```python
from build123d import *

# Parameters (mm, degrees)
SKETCH1_W           = 50.8
SKETCH1_H           = 25.4
BOSS_EXTRUDE1_DEPTH = 6.35
SKETCH2_R           = 3.5
CUT_EXTRUDE1_DEPTH  = 6.35


with BuildPart() as part:
    # Sketch1 → Boss-Extrude1 (new body)
    with BuildSketch(Plane.XY):
        with Locations((25.4, 12.7)):
            Rectangle(SKETCH1_W, SKETCH1_H)
    extrude(amount=BOSS_EXTRUDE1_DEPTH)

    # Sketch2 → Cut-Extrude1 (cut)
    with BuildSketch(Plane.XY.offset(6.35)):
        with Locations((12.7, 12.7)):
            Circle(SKETCH2_R)
        with Locations((38.1, 12.7)):
            Circle(SKETCH2_R)
    extrude(amount=-CUT_EXTRUDE1_DEPTH, mode=Mode.SUBTRACT)


solid = part.part
```
CAD build for the part. Positions are in the model's coordinates, mm. Give positions to 0.01 mm unless a question says otherwise; leave off trailing zeros. Order: outer loops, then holes, each group sorted by start corner. A loop starts at its lowest first (then second) coordinate and runs counter-clockwise, first axis right, second up.
(1) Mould opens along X. For faces 1 (the flat face through (25, 25.4, 3)), 2 (the flat face through (0, 13, 3)), 3 (the cylindrical face through (14.58, 15.65, 3.22)) say: released by +X, released by -X, zero draft, split by the parting line, or undercut.
(2) Saw through at C-C, the plane z = 3. Give the cut face in (x, y).
(3) Saw through at B-B, the plane x = 38.1. Give the cut face in (y, z).
(4) Saw through at D-D, the plane y = 10. Give the cut face in (x, z), then the cut area to 3 significant figures.
(5) Drill centre lines: L1, parallel to X at y = 12.75, z = 5; L2, parallel to Y at x = 38.1, z = 4.25; L3, parallel to Y at x = 10, z = 5.5. Where is each one in solid material? Low to high.
(6) Flat gauge pin, fed straight in: pin 1 (1 mm diameter, centred on x = 25, z = 4, fed in from -Y). Where does the tip first touch, or does it go through?
(7) Saw through at A-A, the plane y = 12.7. Give the cut face in (x, z).
Results found:
1. face 1: zero draft
1. face 2: released by -X
1. face 3: undercut
2. outline: (0, 0) - (50.8, 0) - (50.8, 25.4) - (0, 25.4) - close; hole circle Ø7 at (12.7, 12.7); hole circle Ø7 at (38.1, 12.7)
3. outline: (0, 0) - (9.2, 0) - (9.2, 6.35) - (0, 6.35) - close; (16.2, 0) - (25.4, 0) - (25.4, 6.35) - (16.2, 6.35) - close
4. outline: (0, 0) - (10.47, 0) - (10.47, 6.35) - (0, 6.35) - close; (14.93, 0) - (35.87, 0) - (35.87, 6.35) - (14.93, 6.35) - close; (40.33, 0) - (50.8, 0) - (50.8, 6.35) - (40.33, 6.35) - close
4. area: 266 mm2
5. L1: x = 0 to 9.2, 16.2 to 34.6, 41.6 to 50.8
5. L2: y = 0 to 9.2, 16.2 to 25.4
5. L3: y = 0 to 10.47, 14.93 to 25.4
6. pin 1: stops at y = 0
7. outline: (0, 0) - (9.2, 0) - (9.2, 6.35) - (0, 6.35) - close; (16.2, 0) - (34.6, 0) - (34.6, 6.35) - (16.2, 6.35) - close; (41.6, 0) - (50.8, 0) - (50.8, 6.35) - (41.6, 6.35) - close
